Build history of the part. All positions in model axes, mm. A direction names the side the tool comes from. Round coordinates to 2 decimals unless told otherwise and drop trailing zeros. Loops run counter-clockwise (first coordinate to the right, second up) from the corner with the lowest first, then second, coordinate; pieces in that order, holes last. Notation, with made-up numbers: (5, -40) - (18, -40) arc R24 ccw to (18, -12) - close; hole circle Ø9 at (61, 57.5). An arc over 180 degrees is marked (long way). Use one line per item in the form item = value. Start each with the question number.
Q1. Saw through at C-C (y = 161). Give the cut face in (x, z).
Q2. Saw through at A-A (z = 0). Give the cut face in (x, y).
Q3. Drill centre lines: line 1 (X direction, y = 197.25, z = 0); line 2 (Y direction, x = 0, z = 8); line 3 (Y direction, x = -3.25, z = 2.5). Where is each one in solid material? Low to high.
Q4. Pin check, flat tips, straight feed: pin 1 (3 mm diameter, centred on x = 1.5, y = 128.5, fed in from -Z); pin 2 (4.5 mm diameter, centred on x = 0, z = 0, fed in from +Y); pin 3 (1 mm diameter, centred on x = 5.5, z = -5.5, fed in from -Y). Stop position of each tip, or through.
Q5. Saw through at B-B (x = 0). Give the cut face in (y, z).
Q6. Mould opens along X. For faces 3 (the face through (2.44, -4.93, -0.54)), 4 (the face through (0, -10, 0)), 5 (the face through (0, 192, 0)), 6 (the face through (-2.44, 197.07, -0.54)) say: released by +X, released by -X, zero draft, split by the parting line, or undercut.
Q7. 3-axis set-ups, long thin cutter, end or side, ignore diameter. For faces 1 (the face through (3.2, 201, 10)), 2 (the face through (-2, 0, 2)): which of +Z, -Z, +X, -X, +Y, -Y reach the whole face in a straight line?
```python
from build123d import *

# Parameters (mm, degrees)
SKETCH2_R           = 5
BOSS_EXTRUDE1_DEPTH = 200
SKETCH3_R           = 10.5
BOSS_EXTRUDE2_DEPTH = 2
SKETCH4_R           = 2.5
CUT_EXTRUDE1_DEPTH  = 10
SKETCH5_R           = 2.5
BOSS_EXTRUDE3_DEPTH = 10


with BuildPart() as part:
    # Sketch2 → Boss-Extrude1 (new body)
    with BuildSketch(Plane(origin=(0, 0, 0), x_dir=(1, 0, 0), z_dir=(0, 1, 0))):
        with Locations(Location((0, 0, 0), (0, 0, 270))):
            Circle(SKETCH2_R)
    extrude(amount=BOSS_EXTRUDE1_DEPTH)

    # Sketch3 → Boss-Extrude2 (add)
    with BuildSketch(Plane(origin=(0, 200, 0), x_dir=(1, 0, 0), z_dir=(0, 1, 0))):
        with Locations(Location((0, 0, 0), (0, 0, 270))):
            Circle(SKETCH3_R)
    extrude(amount=BOSS_EXTRUDE2_DEPTH)

    # Sketch4 → Cut-Extrude1 (cut)
    with BuildSketch(Plane(origin=(0, 202, 0), x_dir=(1, 0, 0), z_dir=(0, 1, 0))):
        with Locations(Location((0, 0, 0), (0, 0, 270))):
            Circle(SKETCH4_R)
    extrude(amount=-CUT_EXTRUDE1_DEPTH, mode=Mode.SUBTRACT)

    # Sketch5 → Boss-Extrude3 (add)
    with BuildSketch(Plane.XZ):
        with Locations(Location((0, 0, 0), (0, 0, 90))):
            Circle(SKETCH5_R)
    extrude(amount=BOSS_EXTRUDE3_DEPTH)


solid = part.part
```
Report:
q1.outline = circle Ø10 at (0, 0)
q2.outline = (-10.5, 200) - (-5, 200) - (-5, 0) - (-2.5, 0) - (-2.5, -10) - (2.5, -10) - (2.5, 0) - (5, 0) - (5, 200) - (10.5, 200) - (10.5, 202) - (2.5, 202) - (2.5, 192) - (-2.5, 192) - (-2.5, 202) - (-10.5, 202) - close
q3.line_1 = -5 to -2.5, 2.5 to 5
q3.line_2 = 200 to 202
q3.line_3 = 0 to 202
q4.pin_1 = -5
q4.pin_2 = 192
q4.pin_3 = 200
q5.outline = (-10, -2.5) - (0, -2.5) - (0, -5) - (200, -5) - (200, -10.5) - (202, -10.5) - (202, -2.5) - (192, -2.5) - (192, 2.5) - (202, 2.5) - (202, 10.5) - (200, 10.5) - (200, 5) - (0, 5) - (0, 2.5) - (-10, 2.5) - close
q6.face_3 = split by the parting line
q6.face_4 = zero draft
q6.face_5 = undercut
q6.face_6 = undercut
q7.face_1 = +Y, -Y
q7.face_2 = -Y
